Source: CAD feature listing. Evaluate the final solid. Frame: model axes, mm. Face numbers are marked on the shaded views. A direction names the side the tool comes from. Give positions to 0.01 mm unless a question says otherwise; leave off trailing zeros. Order: outer loops, then holes, each group sorted by start corner. A loop starts at its lowest first (then second) coordinate and runs counter-clockwise, first axis right, second up. Notation, with made-up numbers: M 71.25,52 L 91.25,52 A11 cw 91.25,73 Z; hole C 30.5,49 d9. An arc over 180 degrees is marked long. Answer as a JSON object with one key per item and string values. Group by question number.
1. Section query A-A (x = 0). Output: boundary loops of the cut face in (y, z).
2. Section query D-D (y = 1.75). Output: boundary loops of the cut face in (x, z), plus the area to 3 significant figures.
3. Set-up query: the marked faces 1, 2 and 3. Return all of +Z, -Z, +X, -X, +Y, -Y with unobstructed straight access to the full face (end or side cutting, diameter ignored); none if empty.
4. Pin query (flat end, axial travel): P1, Ø3.5, axis at x = -0.5, z = 2, coming from the +Y side; P2, Ø4, axis at y = -0.5, z = 3, coming from the -X side; P3, Ø5, axis at x = 6.5, y = -1, coming from the +Z side. Return the tip coordinate at first contact, or that it passes through.
5. Pull-direction query (Z, two-part tool) for the marked faces 4, 5 and 6; classes: +Z half, -Z half, draft (parallel to the pull), parting line (faces both ways), or undercut.
6. Material intervals for L1, parallel to X at y = -2, z = 0; L2, parallel to X at y = 5.05, z = 0; L3, parallel to Y at x = 1.25, z = -2.75, sorted ascending. Write a range as [from, to].
7. Section query B-B (z = 0). Output: boundary loops of the cut face in (x, y).
8. Section query C-C (y = 4.25). Output: boundary loops of the cut face in (x, z).
from build123d import *


with BuildPart() as part:
    # Эскиз1 → Повернуть1 (revolve)
    with BuildSketch(Plane.XY, mode=Mode.PRIVATE) as revolve_1_sk:
        with BuildLine():
            Line((2.5, -4.6), (2.5, 4.6))
            Line((2.5, 4.6), (5.5, 4.6))
            Line((5.5, 4.6), (5.5, 5.2))
            Line((5.5, 5.2), (8.5, 5.2))
            Line((8.5, 5.2), (8.5, 3.636698586))
            ThreePointArc((8.5, 3.636698586), (7.25, 1.2), (8.5, -1.236698586))
            Line((8.5, -1.236698586), (8.5, -2.8))
            Line((8.5, -2.8), (4.3, -2.8))
            Line((4.3, -2.8), (4.3, -4.6))
            Line((4.3, -4.6), (2.5, -4.6))
        make_face()
    revolve(revolve_1_sk.sketch.rotate(Axis((0, 0, 0), (0, 1, 0)), 90), axis=Axis((0, 0, 0), (0, 1, 0)))


solid = part.part
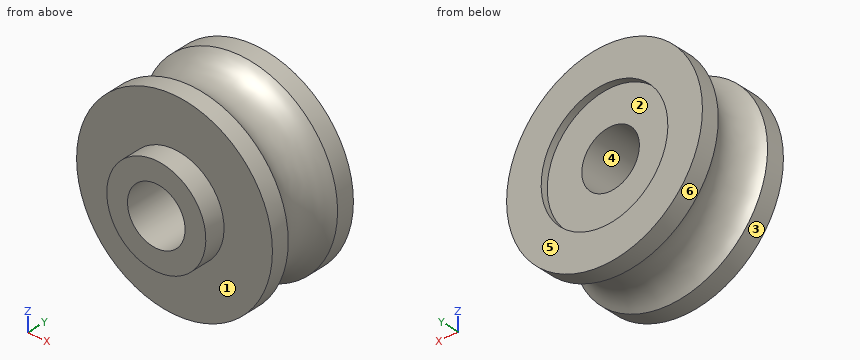
Answer sheet:
{
 "1": {"outline": "M -4.6,-4.3 L -2.8,-4.3 L -2.8,-8.5 L -1.24,-8.5 A3 cw 3.64,-8.5 L 5.2,-8.5 L 5.2,-5.5 L 4.6,-5.5 L 4.6,-2.5 L -4.6,-2.5 Z; M -4.6,2.5 L 4.6,2.5 L 4.6,5.5 L 5.2,5.5 L 5.2,8.5 L 3.64,8.5 A3 cw -1.24,8.5 L -2.8,8.5 L -2.8,4.3 L -4.6,4.3 Z"},
 "2": {"outline": "C 0,0 d14.6; hole C 0,0 d5", "area": "148 mm^2"},
 "3": {"face 1": "-Y", "face 2": "+Y", "face 3": "+Y, -Y"},
 "4": {"P1": "y = 4.6", "P2": "x = -8.42", "P3": "z = 7.49"},
 "5": {"face 4": "undercut", "face 5": "draft", "face 6": "parting line"},
 "6": {"L1": "[-8.5, -2.5], [2.5, 8.5]", "L2": "[-8.5, -5.5], [5.5, 8.5]", "L3": "[-4.6, 4.6]"},
 "7": {"outline": "M -8.5,-2.8 L -4.3,-2.8 L -4.3,-4.6 L -2.5,-4.6 L -2.5,4.6 L -5.5,4.6 L -5.5,5.2 L -8.5,5.2 L -8.5,3.64 A3 cw -8.5,-1.24 Z; M 2.5,-4.6 L 4.3,-4.6 L 4.3,-2.8 L 8.5,-2.8 L 8.5,-1.24 A3 cw 8.5,3.64 L 8.5,5.2 L 5.5,5.2 L 5.5,4.6 L 2.5,4.6 Z"},
 "8": {"outline": "C 0,0 d17; hole C 0,0 d5"}
}
